Could you check a few things on this model? Use its own coordinates, in mm. Face numbers are marked on the shaded views. A direction names the side the tool comes from. Round coordinates to 2 decimals unless told otherwise and drop trailing zeros. Write each loop counter-clockwise with the first axis right and the second up, starting at its lowest first coordinate (ties: lowest second). Pieces come first, ordered by that corner, then holes. Notation, with made-up numbers: (57, 9.25) -> (90, 9.25) arc R38 ccw to (90, 48.25) -> close; hole circle Ø4 at (84, 55.25). An arc over 180 degrees is marked (long way). Return JSON: item names as keys, results as strings.
from build123d import *

# Parameters (mm, degrees)
F1_DEPTH  = 2
F2_R      = 10
F3_DEPTH  = 5
F4_R      = 8
F5_DEPTH  = 4
F6_R      = 3
F7_DEPTH  = 25
F9_DEPTH  = 25
F11_DEPTH = 25
F12_DEPTH = 25


# Not quite as in the source:
# - a feature names something its author has since deleted; it is built from what else it names


with BuildPart() as f1:
    # F0 (on Front) → F1 (new body)
    with BuildSketch(Plane.XZ):
        with BuildLine():
            Line((0, 0), (15.8813624432, -38.3410005992))
            ThreePointArc((15.8813624432, -38.3410005992), (41.5, 0), (15.8813624432, 38.3410005992))
            Line((15.8813624432, 38.3410005992), (0, 0))
        make_face()
        with BuildLine():
            ThreePointArc((0, -41.5), (8.0962483637, -40.7025891367), (15.8813624432, -38.3410005992))
            Line((15.8813624432, -38.3410005992), (0, 0))
            Line((0, 0), (0, -41.5))
        make_face()
        with BuildLine():
            ThreePointArc((15.8813624432, 38.3410005992), (41.5, 0), (15.8813624432, -38.3410005992))
            ThreePointArc((15.8813624432, -38.3410005992), (39.330613444, -23.9742260076), (52.803106606, 0))
            Line((52.803106606, 0), (52.803106606, 36.6300418973))
            Line((52.803106606, 36.6300418973), (100, 73.2887908816))
            Line((100, 73.2887908816), (100, 145.6475704908))
            Line((100, 145.6475704908), (0, 145.6475704908))
            Line((0, 145.6475704908), (-100, 145.6475704908))
            Line((-100, 145.6475704908), (-100, 73.2887908816))
            Line((-100, 73.2887908816), (-52.803106606, 36.6300418973))
            Line((-52.803106606, 36.6300418973), (-52.803106606, 0))
            ThreePointArc((-52.803106606, 0), (-39.330613444, -23.9742260076), (-15.8813624432, -38.3410005992))
            ThreePointArc((-15.8813624432, -38.3410005992), (-41.5, 0), (-15.8813624432, 38.3410005992))
            ThreePointArc((-15.8813624432, 38.3410005992), (0, 41.5), (15.8813624432, 38.3410005992))
        make_face()
        with BuildLine():
            Line((0, -41.5), (0, 0))
            Line((0, 0), (-15.8813624432, -38.3410005992))
            ThreePointArc((-15.8813624432, -38.3410005992), (-8.0962483637, -40.7025891367), (0, -41.5))
        make_face()
        with BuildLine():
            Line((-15.8813624432, -38.3410005992), (0, 0))
            Line((0, 0), (-15.8813624432, 38.3410005992))
            ThreePointArc((-15.8813624432, 38.3410005992), (-41.5, 0), (-15.8813624432, -38.3410005992))
        make_face()
        with BuildLine():
            Line((0, 0), (15.8813624432, 38.3410005992))
            ThreePointArc((15.8813624432, 38.3410005992), (0, 41.5), (-15.8813624432, 38.3410005992))
            Line((-15.8813624432, 38.3410005992), (0, 0))
        make_face()
    extrude(amount=F1_DEPTH)

    # F2 (on face) → F3 (join)
    with BuildSketch(Plane.XZ.offset(2)):
        Circle(F2_R)
    extrude(amount=F3_DEPTH)

    # F4 (on face) → F5 (cut)
    with BuildSketch(Plane(origin=(0, 0, 0), x_dir=(-1, 0, 0), z_dir=(0, 1, 0))):
        Circle(F4_R)
    extrude(amount=-F5_DEPTH, mode=Mode.SUBTRACT)

    # F6 (on face) → F7 (cut)
    with BuildSketch(Plane(origin=(0, 0, 0), x_dir=(-1, 0, 0), z_dir=(0, 1, 0))):
        Circle(F6_R)
    extrude(amount=-F7_DEPTH, mode=Mode.SUBTRACT)

    # F8 (on face) → F9 (join)
    with BuildSketch(Plane.XZ):
        with BuildLine():
            Line((100, 145.6475704908), (94, 145.6475704908))
            Line((94, 145.6475704908), (94, 73.2887908816))
            Line((94, 73.2887908816), (23.1737587601, 37.3859927058))
            ThreePointArc((23.1737587601, 37.3859927058), (38.7897108638, 21.4707349754), (44.803106606, 0))
            Line((44.803106606, 0), (52.803106606, 0))
            Line((52.803106606, 0), (52.803106606, 36.6300418973))
            Line((52.803106606, 36.6300418973), (100, 73.2887908816))
            Line((100, 73.2887908816), (100, 145.6475704908))
        make_face()
        with BuildLine():
            Line((-100, 145.6475704908), (-100, 73.2887908816))
            Line((-100, 73.2887908816), (-52.803106606, 36.6300418973))
            Line((-52.803106606, 36.6300418973), (-52.803106606, 0))
            Line((-52.803106606, 0), (-44.803106606, 0))
            ThreePointArc((-44.803106606, 0), (-38.7897108638, 21.4707349754), (-23.1737587601, 37.3859927058))
            Line((-23.1737587601, 37.3859927058), (-94, 73.2887908816))
            Line((-94, 73.2887908816), (-94, 143.9662277699))
            Line((-94, 143.9662277699), (-94, 145.6475704908))
            Line((-94, 145.6475704908), (-100, 145.6475704908))
        make_face()
    extrude(amount=-F9_DEPTH)

    # F10 (on face) → F11 (join)
    with BuildSketch(Plane.XZ):
        with BuildLine():
            ThreePointArc((44.803106606, 0), (38.1524173859, -20.6793456236), (22.573144677, -35.8171547249))
            ThreePointArc((22.573144677, -35.8171547249), (41.7266336711, -21.3171100871), (52.803106606, 0))
            Line((52.803106606, 0), (44.803106606, 0))
        make_face()
    extrude(amount=-F11_DEPTH)

    # F10 (on face) → F12 (join)
    with BuildSketch(Plane.XZ):
        with BuildLine():
            ThreePointArc((-52.803106606, 0), (-41.7266336711, -21.3171100871), (-22.573144677, -35.8171547249))
            ThreePointArc((-22.573144677, -35.8171547249), (-38.1524173859, -20.6793456236), (-44.803106606, 0))
            Line((-44.803106606, 0), (-52.803106606, 0))
        make_face()
    extrude(amount=-F12_DEPTH)


solid = f1.part
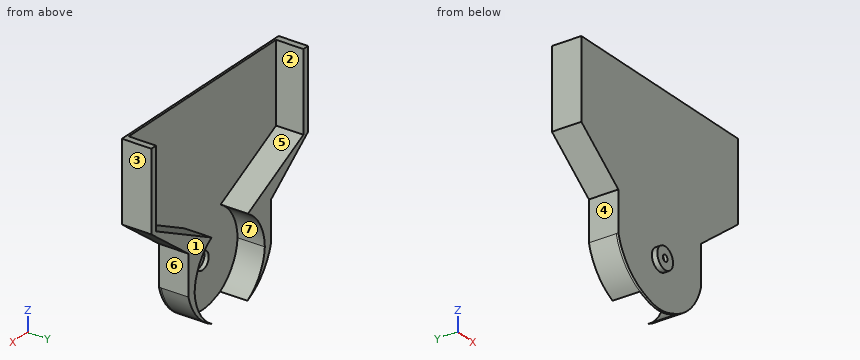
1) I want a section at B-B, the plane z = 71. Please give me the cut outline in (x, y), and give its area (3 significant figures).
Return value:
{"outline": "(-97.05, -2) -> (97.05, -2) -> (97.05, 25) -> (89.48, 25) -> (89.48, 0) -> (-89.48, 0) -> (-89.48, 25) -> (-97.05, 25) -> close", "area": "767 mm²"}
2) Thinking about a two-plate mould opening in X: for the marked faces 1, 2 and 3, which applies, pulls with the +X half, pulls with the -X half, needs draft (parallel to the pull), parting line crosses it, or undercut?
Return value:
{"face 1": "needs draft", "face 2": "undercut", "face 3": "pulls with the +X half"}
3) I want a section at C-C, the plane x = -35. Please give me the cut outline in (y, z), and give its area (3 significant figures).
Return value:
{"outline": "(-2, -28.01) -> (25, -28.01) -> (25, -25.13) -> (0, -25.13) -> (0, 27.02) -> (25, 27.02) -> (25, 43.38) -> (0, 43.38) -> (0, 145.65) -> (-2, 145.65) -> close", "area": "828 mm²"}
4) For the marked faces 4, 5, 6 and 7, which set-ups out of +Z, -Z, +X, -X, +Y, -Y let a thin tool reach every point of the face, with its end or its side?
Return value:
{"face 4": "-Z, -X, +Y, -Y", "face 5": "+Z, +Y", "face 6": "-Z, +X, +Y, -Y", "face 7": "+Y"}
5) Will these pins go through, and if not, where does the flat tip stop? pin 1 Ø2 at (x, z) = (24, 83) entering from -Y; pin 2 Ø8 at (y, z) = (-2.5, 39) entering from -X; pin 3 Ø13 at (x, z) = (3, -1) entering from +Y.
Return value:
{"pin 1": "y = -2", "pin 2": "x = -60.96", "pin 3": "y = 0"}
6) If I drill on probe 1 along X at (y, z) = (16, 103); probe 2 along Z at (x, y) = (0, -2.5); probe 3 along Z at (x, y) = (0, -5.7), over which ranges is the centre line in solid material (lowest first)? Write a range as [from, to].
Return value:
{"probe 1": "[-100, -94], [94, 100]", "probe 2": "[-10, -8], [8, 10]", "probe 3": "[-10, -3], [3, 10]"}
7) I want a section at D-D, the plane x = 78.5. Please give me the cut outline in (y, z), and give its area (3 significant figures).
Return value:
{"outline": "(-2, 56.59) -> (25, 56.59) -> (25, 65.43) -> (0, 65.43) -> (0, 145.65) -> (-2, 145.65) -> close", "area": "399 mm²"}
8) I want a section at A-A, the plane y = 21. Please give me the cut outline in (x, z), and give its area (3 significant figures).
Return value:
{"outline": "(-100, 73.29) -> (-52.8, 36.63) -> (-52.8, 0) arc R54.6 ccw to (-22.57, -35.82) arc R44.9 cw to (-44.8, 0) arc R44.81 cw to (-23.17, 37.39) -> (-94, 73.29) -> (-94, 145.65) -> (-100, 145.65) -> close; (22.57, -35.82) arc R54.6 ccw to (52.8, 0) -> (52.8, 36.63) -> (100, 73.29) -> (100, 145.65) -> (94, 145.65) -> (94, 73.29) -> (23.17, 37.39) arc R44.81 cw to (44.8, 0) arc R44.9 cw to start", "area": "3,590 mm²"}
